Verification items for this drawing (mm, ordinates from the low corner). Coordinates: 2 decimals unless noted, no trailing zeros. Write each loop counter-clockwise with the first axis right and the second up, starting at its lowest first coordinate (ties: lowest second). Pieces come first, ordered by that corner, then holes. Notation, with made-up numbers: M 8,57.25 L 45,57.25 A8 cw 45,68.25 Z; hole C 57.25,21 d8. An arc over 180 degrees is marked long. Put each result on its own line as item: value. Start each with the question number.
1) Scan lines: line 1 along Y through (x, z) = (14, 5.25); line 2 along X through (y, z) = (2, 6.25); line 3 along X through (y, z) = (9.75, 3.5). Record each from-to range of solid material in increasing order.
2) Cross-section at D-D on y = 0.5. Record the cut outline in (x, z).
3) Mould release check, pull along X, two halves, no side actions. Record for the marked faces 1, 2, 3 and 4: released by +X, released by -X, zero draft, split by the parting line, or undercut.
4) Cross-section at A-A on z = 5. Record the cut outline in (x, y).
5) Cross-section at C-C on x = 14. Record the cut outline in (y, z).
6) Cross-section at B-B on y = 5. Record the cut outline in (x, z).
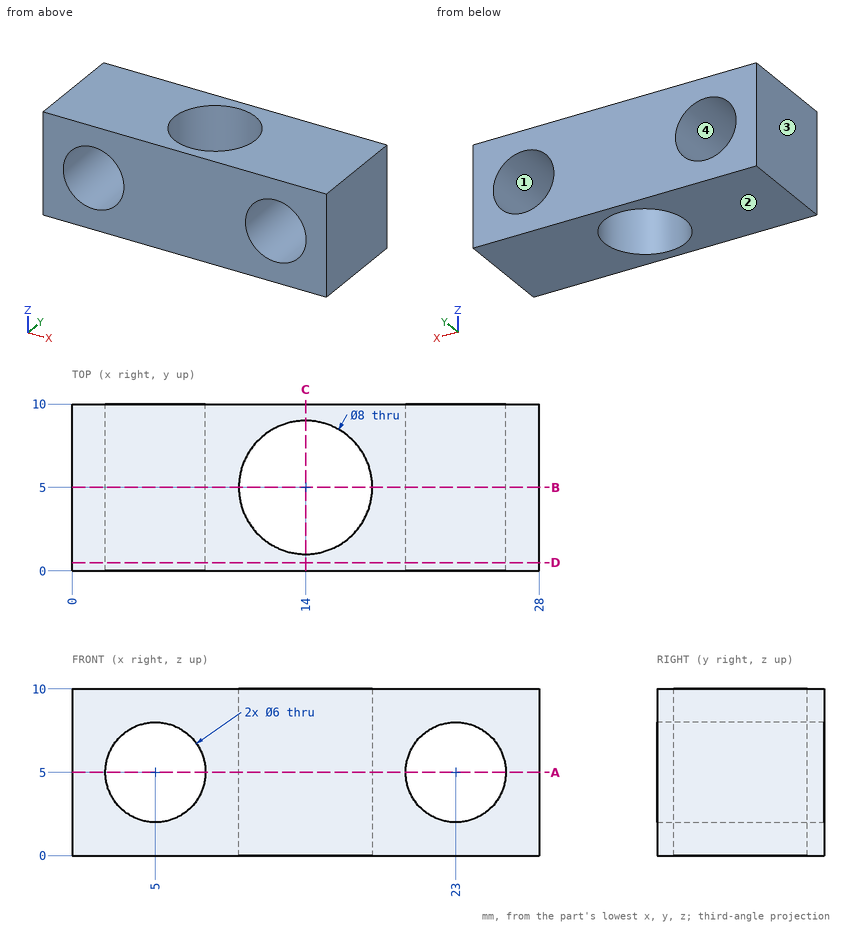
Answer key:
1. line 1: y = 0 to 1, 9 to 10
1. line 2: x = 0 to 2.27, 7.73 to 11.35, 16.65 to 20.27, 25.73 to 28
1. line 3: x = 0 to 2.4, 7.6 to 20.4, 25.6 to 28
2. outline: M 0,0 L 28,0 L 28,10 L 0,10 Z; hole C 5,5 d6; hole C 23,5 d6
3. face 1: undercut
3. face 2: zero draft
3. face 3: released by -X
3. face 4: undercut
4. outline: M 0,0 L 2,0 L 2,10 L 0,10 Z; M 8,0 L 20,0 L 20,10 L 8,10 Z; M 26,0 L 28,0 L 28,10 L 26,10 Z; hole C 14,5 d8
5. outline: M 0,0 L 1,0 L 1,10 L 0,10 Z; M 9,0 L 10,0 L 10,10 L 9,10 Z
6. outline: M 0,0 L 10,0 L 10,10 L 0,10 Z; M 18,0 L 28,0 L 28,10 L 18,10 Z; hole C 5,5 d6; hole C 23,5 d6
